Geometry check sheet. Reference: drawing and pictorial views, mm from the part's lowest x, y, z. A direction names the side the tool comes from. Coordinates: 2 decimals unless noted, no trailing zeros. Loops run counter-clockwise (first coordinate to the right, second up) from the corner with the lowest first, then second, coordinate; pieces in that order, holes last. Notation, with made-up numbers: (78, 83.5) -> (121, 83.5) arc R16 ccw to (121, 104.5) -> close; hole circle Ø6 at (51, 13.5). An arc over 180 degrees is marked (long way). Answer as a JSON object with one key per item and string values.
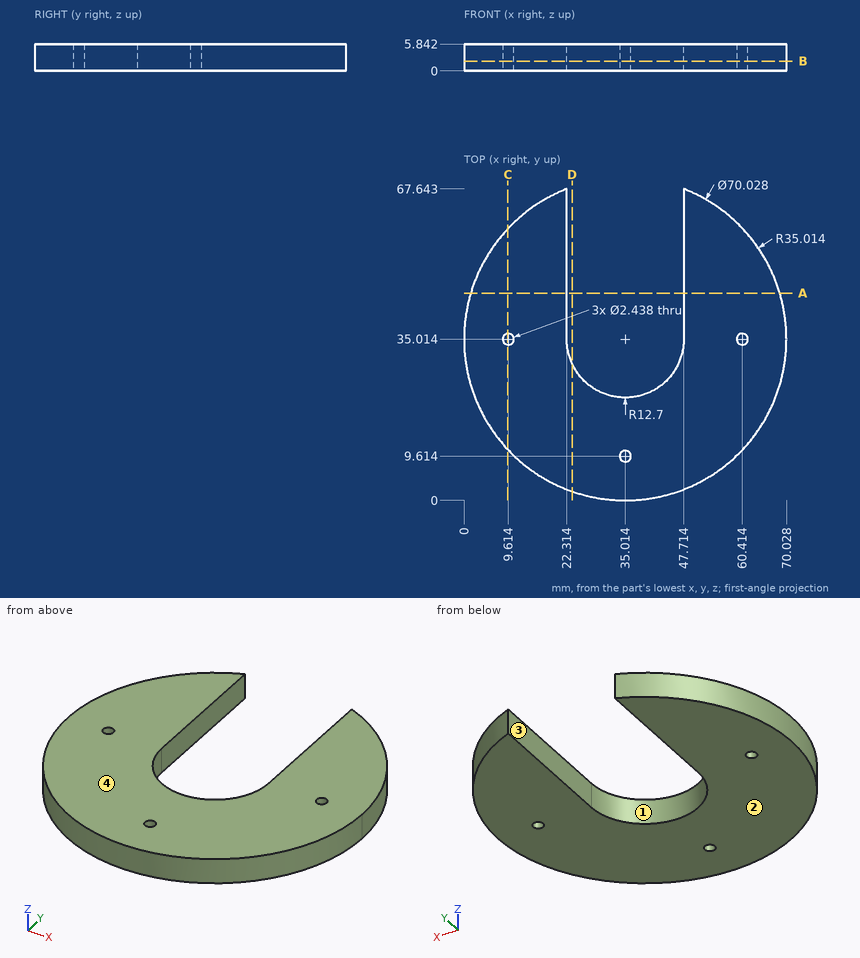
1. Thickness scan on probe 1 along X at (y, z) = (36, 4.35) (1 decimal); probe 2 along X at (y, z) = (49, 3.05) (1 decimal); probe 3 along X at (y, z) = (60.5, 2.1) (1 decimal). Record the ranges inside material, lowest first. Write a range as from..to.
Evaluation:
{"probe 1": "x = 0..8.9, 10.3..22.3, 47.7..59.7, 61.1..70", "probe 2": "x = 2.9..22.3, 47.7..67.1", "probe 3": "x = 11..22.3, 47.7..59"}
2. Tool access check on the marked faces 3 and 4. Record the directions out of +Z, -Z, +X, -X, +Y, -Y that give a thin tool (end or side, any length) a straight path to the whole face; none if there is none.
Evaluation:
{"face 3": "+Z, -Z, +Y", "face 4": "+Z, +X, -X, +Y, -Y"}
3. Mould release check, pull along X, two halves, no side actions. Record for the marked faces 1 and 2: released by +X, released by -X, zero draft, split by the parting line, or undercut.
Evaluation:
{"face 1": "undercut", "face 2": "zero draft"}
4. Section check B-B, the plane z = 2.15. Record the boundary of the cut face in (x, y), then the cut area to 3 significant figures.
Evaluation:
{"outline": "(22.31, 35.01) -> (22.31, 67.64) arc R35.01 ccw (long way) to (47.71, 67.64) -> (47.71, 35.01) arc R12.7 cw to start; hole circle Ø2.44 at (9.61, 35.01); hole circle Ø2.44 at (35.01, 9.61); hole circle Ø2.44 at (60.41, 35.01)", "area": "2,710 mm^2"}
5. Section check D-D, the plane x = 23.5. Record the boundary of the cut face in (y, z) (1 decimal).
Evaluation:
{"outline": "(1.9, 0) -> (29.7, 0) -> (29.7, 5.8) -> (1.9, 5.8) -> close"}
6. Section check A-A, the plane y = 45. Record the boundary of the cut face in (x, z) (1 decimal).
Evaluation:
{"outline": "(1.5, 0) -> (22.3, 0) -> (22.3, 5.8) -> (1.5, 5.8) -> close; (47.7, 0) -> (68.6, 0) -> (68.6, 5.8) -> (47.7, 5.8) -> close"}
7. Section check C-C, the plane x = 9.5. Record the boundary of the cut face in (y, z) (1 decimal), then the cut area to 3 significant figures.
Evaluation:
{"outline": "(11, 0) -> (33.8, 0) -> (33.8, 5.8) -> (11, 5.8) -> close; (36.2, 0) -> (59, 0) -> (59, 5.8) -> (36.2, 5.8) -> close", "area": "266 mm^2"}
8. Depth check by flat-ended pin: P1, Ø1, axis at x = 38, z = 1, coming from the +Y side; P2, Ø3, axis at x = 62, z = 4, coming from the -Y side (1 decimal); P3, Ø3, axis at y = 43, z = 2.5, coming from the +X side. Enter the tip coordinate at first touch or a pass-through.
Evaluation:
{"P1": "stops at y = 22.8", "P2": "stops at y = 11", "P3": "stops at x = 69.42"}
